Design review of the part built by this model. Coordinates are the model's own, in mm. A direction names the side the tool comes from. Coordinates: 2 decimals unless noted, no trailing zeros. Order: outer loops, then holes, each group sorted by start corner. A loop starts at its lowest first (then second) coordinate and runs counter-clockwise, first axis right, second up. Notation, with made-up numbers: (-39, 46) -> (-18, 46) arc R16 ccw to (-18, 55) -> close; hole circle Ø2 at (60, -9.5). An arc over 180 degrees is marked (long way). Write item = value, one per line.
Autodesk Inventor part; units mm, degrees
ref_plane "YZ Plane" through (0, 0, 0) normal (1, 0, 0) x (0, 1, 0)
ref_plane "XZ Plane" through (0, 0, 0) normal (0, 1, 0) x (-1, 0, 0)
ref_plane "XY Plane" through (0, 0, 0) normal (0, 0, 1) x (1, 0, 0)
sketch "Sketch1" plane through (0, 0, 0) normal (0, 0, 1) x (1, 0, 0)
  arc A0 (18.8782, 11.9777) -> (7.1013, 4.6885) centre (18.1475, 0) ccw
  arc A1 (18.8782, 11.9777) -> (21, 13.974) centre (19, 13.974) ccw
  line L0 (21, 13.974) -> (21, 19)
  arc A2 (21, 19) -> (19, 21) centre (19, 19) ccw
  line L1 (19, 21) -> (-19, 21)
  arc A3 (-19, 21) -> (-21, 19) centre (-19, 19) ccw
  line L2 (-21, 19) -> (-21, -19)
  arc A4 (-21, -19) -> (-19, -21) centre (-19, -19) ccw
  line L3 (-19, -21) -> (7.9725, -21)
  arc A5 (9.9725, -23) -> (7.9725, -21) centre (7.9725, -23) ccw
  line L4 (9.9725, -23.6) -> (9.9725, -23)
  arc A6 (9.9725, -23.6) -> (11.9725, -25.6) centre (11.9725, -23.6) ccw
  line L5 (19, -25.6) -> (11.9725, -25.6)
  arc A7 (19, -25.6) -> (21, -23.6) centre (19, -23.6) ccw
  line L6 (21, -13.974) -> (21, -23.6)
  arc A8 (21, -13.974) -> (18.8782, -11.9777) centre (19, -13.974) ccw
  circle A9 centre (-15.5, 15.5) radius 1.6
  circle A10 centre (15.5, -15.5) radius 1.6
  circle A11 centre (-15.5, -15.5) radius 1.6
  circle A12 centre (15.5, 15.5) radius 1.6
  arc A13 (21, 19) -> (19, 21) centre (19, 19) ccw
  line L7 (21, 13.974) -> (21, 19)
  arc A14 (18.8782, 11.9777) -> (21, 13.974) centre (19, 13.974) ccw
  arc A15 (18.8782, 11.9777) -> (9, 7.7668) centre (18.1475, 0) ccw
  line L8 (9, 7.7668) -> (9, 19)
  arc A16 (9, 19) -> (7, 21) centre (7, 19) ccw
  line L9 (19, 21) -> (7, 21)
  circle A17 centre (15.5, 15.5) radius 1.6
  arc A18 (15.5, 18.5) -> (12.5, 15.5) centre (15.5, 15.5) ccw
  arc A19 (12.5, 0) -> (18.1475, -5.6475) centre (18.1475, 0) ccw
  line L10 (12.5, 15.5) -> (12.5, 0)
  line L11 (18.1475, -5.6475) -> (26, -5.6475)
  line L12 (26, -5.6475) -> (26, -31.6)
  line L13 (26, -31.6) -> (33.5, -31.6)
  line L14 (33.5, -31.6) -> (33.5, 18.5)
  line L15 (33.5, 18.5) -> (15.5, 18.5)
  arc A20 (5.4082, 4.4443) -> (7.1013, 4.6885) centre (6.1808, 5.0792) ccw
  arc A21 (7.1013, -4.6885) -> (18.8782, -11.9777) centre (18.1475, 0) ccw
  arc A22 (7.1013, -4.6885) -> (5.4082, -4.4443) centre (6.1808, -5.0792) ccw
  arc A23 (5.4082, 4.4443) -> (5.4082, -4.4443) centre (0, 0) ccw
  point P0 (0, 0)
  point P1 (29.75, -31.6)
  dimension "d1" = 7.5
  dimension "d2" = 5
  dimension "d3" = 6
  dimension "d39" = 3
extrude "Extrusion1" add sketch "Sketch1" along normal blind 22 contours L10 A18 L15 L0 A1 A0 | A0 A1 L0 L15 L14 L13 L12 L11 A19 L10
sketch "Sketch2" plane through (0, 0, 22) normal (0, 0, 1) x (1, 0, 0)
  circle A0 centre (15.5, 15.5) radius 1.6
  arc A1 (15.5, 18.5) -> (12.5, 15.5) centre (15.5, 15.5) ccw
  circle A2 centre (15.5, 15.5) radius 7.5
  point P0 (0, 0)
  dimension "d6" = 15
extrude "Extrusion2" cut sketch "Sketch2" against normal blind 4.5
ref_plane "Work Plane1" through (0, 0, 11) normal (0, 0, 1) x (1, 0, 0)
sketch "Sketch3" plane through (0, 0, 11) normal (0, 0, 1) x (1, 0, 0)
  line L0 (15.5, 18.5) -> (33.5, 18.5)
  line L1 (33.5, 18.5) -> (33.5, -31.6)
  line L2 (33.5, -31.6) -> (26, -31.6)
  line L3 (26, -31.6) -> (26, -5.6475)
  line L4 (26, -5.6475) -> (18.1475, -5.6475)
  arc A0 (12.5, 0) -> (18.1475, -5.6475) centre (18.1475, 0) ccw
  line L5 (12.5, 0) -> (12.5, 15.5)
  arc A1 (15.5, 18.5) -> (12.5, 15.5) centre (15.5, 15.5) ccw
  circle A2 centre (15.5, 15.5) radius 1.6
  circle A3 centre (18.1475, 0) radius 12.5
  point P0 (0, 0)
  dimension "d11" = 25
extrude "Extrusion3" cut sketch "Sketch3" along normal mid plane 9 contours A3 L3 L4 A0 L5 | L5 A0 L4 L3 A3
sketch "Sketch4" plane through (0, 0, 6.5) normal (0, 0, 1) x (1, 0, 0)
  arc A0 (12.5, 0) -> (18.1475, -5.6475) centre (18.1475, 0) ccw
  arc A1 (26, -9.7256) -> (12.5, 11.1515) centre (18.1475, 0) ccw
  circle A2 centre (18.1475, 0) radius 5.6475
  point P0 (0, 0)
extrude "Extrusion4" add sketch "Sketch4" along normal blind 0.9 draft -45
mirror "Mirror1" about plane through (0, 0, 11) normal (0, 0, 1) of "Extrusion4"
sketch "Sketch5" plane through (0, 0, 22) normal (0, 0, 1) x (1, 0, 0)
  arc A0 (12.5, 0) -> (18.1475, -5.6475) centre (18.1475, 0) ccw
  circle A1 centre (18.1475, 0) radius 1.6
  point P0 (0, 0)
  dimension "d18" = 3.2
extrude "Extrusion5" cut sketch "Sketch5" against normal through all
sketch "Sketch6" plane through (0, 0, 0) normal (0, 0, -1) x (-1, 0, 0)
  circle A0 centre (-18.1475, 0) radius 1.6
  arc A1 (-18.1475, -5.6475) -> (-12.5, 0) centre (-18.1475, 0) ccw
  circle A2 centre (-18.1475, 0) radius 3
  point P0 (0, 0)
  dimension "d23" = 6
extrude "Extrusion6" cut sketch "Sketch6" against normal blind 3
sketch "Sketch7" plane through (0, 0, 22) normal (0, 0, 1) x (1, 0, 0)
  circle A0 centre (18.1475, 0) radius 1.6
  arc A1 (12.5, 0) -> (18.1475, -5.6475) centre (18.1475, 0) ccw
  line L0 (18.1475, 3.262) -> (20.9725, 1.631)
  line L1 (20.9725, 1.631) -> (20.9725, -1.631)
  line L2 (20.9725, -1.631) -> (18.1475, -3.262)
  line L3 (18.1475, -3.262) -> (15.3225, -1.631)
  line L4 (15.3225, -1.631) -> (15.3225, 1.631)
  line L5 (15.3225, 1.631) -> (18.1475, 3.262)
  point P0 (0, 0)
  dimension "d27" = 5.65
extrude "Extrusion7" cut sketch "Sketch7" against normal blind 2.5
sketch "Sketch8" plane through (33.5, -31.6, 0) normal (1, 0, 0) x (0, 0, -1)
  line L0 (-22, 17.626) -> (0, 17.626)
  line L1 (-17.2286, 8) -> (-22, 8)
  arc A0 (-14.7539, 10.0285) -> (-17.2286, 8) centre (-15.9796, 9) ccw
  line L2 (-14.7539, 10.0285) -> (-13.0518, 8)
  line L3 (-7.2286, 8) -> (-13.0518, 8)
  arc A1 (-4.7539, 10.0285) -> (-7.2286, 8) centre (-5.9796, 9) ccw
  line L4 (-4.7539, 10.0285) -> (-3.0518, 8)
  line L5 (0, 8) -> (-3.0518, 8)
  line L6 (0, 17.626) -> (0, 8)
  line L7 (-13.0518, 8) -> (-12.2843, 7.0853)
  arc A2 (-14.7353, 5.0287) -> (-12.2843, 7.0853) centre (-13.5098, 6.057) ccw
  line L8 (-14.7353, 5.0287) -> (-17.2286, 8)
  line L9 (-3.0518, 8) -> (-2.2607, 7.0571)
  arc A3 (-4.8043, 4.9721) -> (-2.2607, 7.0571) centre (-3.5205, 6) ccw
  line L10 (-4.8043, 4.9721) -> (-7.2286, 8)
  line L11 (-22, 17.626) -> (-22, 8)
  point P0 (0, 31.6)
  dimension "d30" = 3
extrude "Extrusion8" cut sketch "Sketch8" against normal through all contours A0 L2 L7 A2 L8 | L9 A3 L10 A1 L4
sketch "Sketch9" plane through (33.5, -31.6, 0) normal (1, 0, 0) x (0, 0, -1)
  line L0 (-4.7539, 10.0285) -> (-2.2607, 7.0571)
  line L1 (0, 50.1) -> (0, 0)
  line L2 (-22, 0) -> (-22, 50.1)
  line L3 (0, 0) -> (-22, 0)
  line L4 (0, 1.057) -> (-13.5098, 1.057)
  arc A0 (-17.3401, 2.8431) -> (-13.5098, 1.057) centre (-13.5098, 6.057) ccw
  line L5 (-17.3401, 2.8431) -> (-22, 8.3966)
  arc A1 (-14.7353, 5.0287) -> (-12.2843, 7.0853) centre (-13.5098, 6.057) ccw
  point P0 (0, 31.6)
  dimension "d33" = 5
extrude "Extrusion9" cut sketch "Sketch9" against normal through all
fillet "Fillet1" radius 3 8 edges at (26, -5.6475, 18.75) (26, -5.6475, 3.25) (12.5, 11.1515, 11) (26, -9.7256, 11) (29.75, -23.2034, 22) (29.75, -30.543, 0) (12.5, 8.6261, 19.75) (22.3739, 18.5, 19.75)
properties part number "ARM"
(1) We need section B-B (z = 4.25). Write out the cut boundary in (x, y) (1 decimal).
Report:
outline = (12.5, 0) arc R5.6 ccw to (18.1, -5.6) -> (23, -5.6) arc R3 cw to (26, -8.6) -> (26, -22.2) -> (33.5, -22.2) -> (33.5, 18.5) -> (15.5, 18.5) arc R3 ccw to (12.5, 15.5) -> close; (26, -30.5) -> (33.5, -30.5) -> (33.5, -27.1) -> (26, -27.1) -> close; hole circle Ø3.2 at (15.5, 15.5); hole circle Ø3.2 at (18.1, 0)
(2) For faces 4 (the cylindrical face through (26.24, -9.89, 11.06)), 5 (the flat face through (29.8, -25.11, 15.96)), 6 (the flat face through (20, 0, 7.4)), list the 3-axis set-ups (+Z, -Z, +X, -X, +Y, -Y) from which the entire face can be reached by the end or side of a thin tool; tool diameter is ignored.
Report:
face_4 = -X
face_5 = +X, -X
face_6 = -X, -Y
(3) We need section D-D (x = 24.5). Write out the cut boundary in (y, z), and give its area (3 significant figures).
Report:
outline = (-6.05, 0) -> (18.5, 0) -> (18.5, 17.5) -> (18.1, 17.5) -> (18.1, 22) -> (-6.05, 22) -> (-6.05, 15.5) -> (10.77, 15.5) -> (10.77, 6.5) -> (-6.05, 6.5) -> close
area = 387 mm²
(4) For L1, parallel to Z at x = 15.5, y = 11; L2, parallel to Y at x = 16.25, z = 14.75; L3, parallel to Z at x = 18.25, y = 6, list the stretches that pass through material, from the lowest coordinate up.
Report:
L1 = 0 to 6.5, 15.5 to 17.5
L2 = -4.51 to 4.51, 12.36 to 14.09, 16.91 to 18.5
L3 = 0 to 6.5, 15.5 to 22
(5) The part is to be moulded in two halves that separate along X. For faces 1 (the flat face through (20.972, 0, 21)), 2 (the flat face through (21, -5.648, 19)), 3 (the flat face through (26, -19, 11)), say which applies: released by +X, released by -X, zero draft, split by the parting line, or undercut.
Report:
face_1 = undercut
face_2 = zero draft
face_3 = released by -X
(6) Insertion check: pin 1 (5.5 mm diameter, centred on x = 18.15, y = 0, fed in from -Z); pin 2 (5.5 mm diameter, centred on x = 19.5, z = 3.5, fed in from -Y); pin 3 (5.5 mm diameter, centred on x = 21.5, z = 18.5, fed in from -Y); pin 4 (2.5 mm diameter, centred on x = 18.15, y = 0, fed in from -Z). Each pin has a flat end and moves straight along its axis. Give the tip position at first contact, or say it passes through.
Report:
pin_1 = 3
pin_2 = -5.65
pin_3 = -5.92
pin_4 = through
(7) We need section C-C (y = 6.5). Write out the cut boundary in (x, z).
Report:
outline = (12.5, 0) -> (33.5, 0) -> (33.5, 22) -> (12.9, 22) -> (12.9, 17.5) -> (12.5, 17.5) -> (12.5, 15.5) -> (28.82, 15.5) -> (28.82, 6.5) -> (12.5, 6.5) -> close
(8) We need section A-A (x = 29.75). Write out the cut boundary in (y, z), and give its area (3 significant figures).
Report:
outline = (-30.54, 3) arc R3 ccw to (-27.54, 0) -> (18.5, 0) -> (18.5, 22) -> (-22.11, 22) arc R3 ccw to (-24.04, 21.3) -> (-28.76, 17.34) arc R5 ccw to (-30.54, 13.51) -> close; hole (-26.63, 4.8) arc R1.64 ccw (long way) to (-24.54, 2.26) -> (-23.6, 3.05) -> (-21.57, 4.75) arc R1.6 ccw to (-23.6, 7.23) -> close; hole (-26.57, 14.74) arc R1.6 ccw to (-24.51, 12.28) -> (-23.6, 13.05) -> (-21.57, 14.75) arc R1.6 ccw to (-23.6, 17.23) -> close; hole (-4.65, 6.5) -> (4.65, 6.5) -> (4.65, 15.5) -> (-4.65, 15.5) -> close
area = 929 mm²
